For this review, take the finished solid that the model builds, in its own axes (mm). Face numbers are marked on the shaded views. Round coordinates to 2 decimals unless told otherwise and drop trailing zeros. Order: outer loops, then holes, each group sorted by start corner. A loop starts at its lowest first (then second) coordinate and runs counter-clockwise, first axis right, second up. Notation, with made-up numbers: (22, 72.25) - (49, 72.25) arc R12 ccw to (49, 93.25) - close; hole circle Ø4 at (8.5, 84). An arc over 180 degrees is marked (long way). One line per item, written item: value.
```python
from build123d import *

# Parameters (mm, degrees)
SPUR_START             = -54.751290346
SPUR_GEAR_AI_OUTLINE_R = 4.7625
SPUR_GEAR_AI_DEPTH     = 11.684
CUT_EXTRUDE1_DEPTH     = 45.73825268


# Read off the part's stored shape, not the designer's step: spur gear_ai
with BuildPart() as part:
    # spur gear_ai outline → spur gear_ai (new body)
    with BuildSketch(Plane.YZ.offset(SPUR_START)):
        with BuildLine():
            ThreePointArc((6.265843754, 23.742611923), (6.505460201, 24.059955507), (6.73322633, 24.385908852))
            ThreePointArc((6.73322633, 24.385908852), (5.912883536, 25.630805773), (4.677624003, 26.465589895))
            ThreePointArc((4.677624003, 26.465589895), (5.034990844, 27.171459646), (5.320429206, 27.90935402))
            ThreePointArc((5.320429206, 27.90935402), (6.767344667, 27.549956895), (8.241399844, 27.773322024))
            ThreePointArc((8.241399844, 27.773322024), (8.331225097, 28.160690604), (8.40672264, 28.551104632))
            ThreePointArc((8.40672264, 28.551104632), (7.150957012, 29.354711085), (5.682953985, 29.614899012))
            ThreePointArc((5.682953985, 29.614899012), (5.722321747, 30.405097306), (5.682953985, 31.1952956))
            ThreePointArc((5.682953985, 31.1952956), (7.150957012, 31.455483527), (8.40672264, 32.25908998))
            ThreePointArc((8.40672264, 32.25908998), (8.331225097, 32.649504008), (8.241399844, 33.036872588))
            ThreePointArc((8.241399844, 33.036872588), (6.767344667, 33.260237716), (5.320429206, 32.900840592))
            ThreePointArc((5.320429206, 32.900840592), (5.034990844, 33.638734965), (4.677624003, 34.344604716))
            ThreePointArc((4.677624003, 34.344604716), (5.912883536, 35.179388839), (6.73322633, 36.42428576))
            ThreePointArc((6.73322633, 36.42428576), (6.505460201, 36.750239104), (6.265843754, 37.067582688))
            ThreePointArc((6.265843754, 37.067582688), (4.82837656, 36.672084633), (3.652733492, 35.755245485))
            ThreePointArc((3.652733492, 35.755245485), (3.091843894, 36.313247297), (2.478269946, 36.812737212))
            ThreePointArc((2.478269946, 36.812737212), (3.26719839, 38.077775771), (3.510273629, 39.548709173))
            ThreePointArc((3.510273629, 39.548709173), (3.169621747, 39.75384154), (2.821645965, 39.94628854))
            ThreePointArc((2.821645965, 39.94628854), (1.669317892, 39.000312507), (0.968226585, 37.684561153))
            ThreePointArc((0.968226585, 37.684561153), (0.228868656, 37.966186822), (-0.534819889, 38.172930557))
            ThreePointArc((-0.534819889, 38.172930557), (-0.328635429, 39.649486893), (-0.704857663, 41.092119028))
            ThreePointArc((-0.704857663, 41.092119028), (-1.099493493, 41.140961166), (-1.495660434, 41.175235748))
            ThreePointArc((-1.495660434, 41.175235748), (-2.163601395, 39.842349587), (-2.268915885, 38.35519139))
            ThreePointArc((-2.268915885, 38.35519139), (-3.058900442, 38.311745278), (-3.840654895, 38.189994964))
            ThreePointArc((-3.840654895, 38.189994964), (-4.252865586, 39.622759072), (-5.18333305, 40.787645738))
            ThreePointArc((-5.18333305, 40.787645738), (-5.563716707, 40.671752399), (-5.939573945, 40.541928176))
            ThreePointArc((-5.939573945, 40.541928176), (-6.007634734, 39.052600014), (-5.498962575, 37.651178136))
            ThreePointArc((-5.498962575, 37.651178136), (-6.202978253, 37.290172471), (-6.867626169, 36.860979842))
            ThreePointArc((-6.867626169, 36.860979842), (-7.826957037, 38.002213793), (-9.150783454, 38.687935502))
            ThreePointArc((-9.150783454, 38.687935502), (-9.451143149, 38.427345697), (-9.741701553, 38.155870456))
            ThreePointArc((-9.741701553, 38.155870456), (-9.19811384, 36.767618662), (-8.16340907, 35.694251677))
            ThreePointArc((-8.16340907, 35.694251677), (-8.659725162, 35.078107619), (-9.092342877, 34.41568398))
            ThreePointArc((-9.092342877, 34.41568398), (-10.4329169, 35.068058055), (-11.921200656, 35.156047294))
            ThreePointArc((-11.921200656, 35.156047294), (-12.089601468, 34.795819368), (-12.24462085, 34.429633645))
            ThreePointArc((-12.24462085, 34.429633645), (-11.18337589, 33.382499566), (-9.801548363, 32.822782378))
            ThreePointArc((-9.801548363, 32.822782378), (-10.004347308, 32.05803683), (-10.13013129, 31.276921247))
            ThreePointArc((-10.13013129, 31.276921247), (-11.62015104, 31.327634041), (-13.015554353, 30.802676673))
            ThreePointArc((-13.015554353, 30.802676673), (-13.022878253, 30.405097306), (-13.015554353, 30.007517939))
            ThreePointArc((-13.015554353, 30.007517939), (-11.62015104, 29.48256057), (-10.13013129, 29.533273365))
            ThreePointArc((-10.13013129, 29.533273365), (-10.004347308, 28.752157782), (-9.801548363, 27.987412234))
            ThreePointArc((-9.801548363, 27.987412234), (-11.18337589, 27.427695046), (-12.24462085, 26.380560967))
            ThreePointArc((-12.24462085, 26.380560967), (-12.089601468, 26.014375244), (-11.921200656, 25.654147317))
            ThreePointArc((-11.921200656, 25.654147317), (-10.4329169, 25.742136557), (-9.092342877, 26.394510632))
            ThreePointArc((-9.092342877, 26.394510632), (-8.659725162, 25.732086993), (-8.16340907, 25.115942934))
            ThreePointArc((-8.16340907, 25.115942934), (-9.19811384, 24.04257595), (-9.741701553, 22.654324156))
            ThreePointArc((-9.741701553, 22.654324156), (-9.451143149, 22.382848915), (-9.150783454, 22.12225911))
            ThreePointArc((-9.150783454, 22.12225911), (-7.826957037, 22.807980819), (-6.867626169, 23.94921477))
            ThreePointArc((-6.867626169, 23.94921477), (-6.202978253, 23.520022141), (-5.498962575, 23.159016476))
            ThreePointArc((-5.498962575, 23.159016476), (-6.007634734, 21.757594598), (-5.939573945, 20.268266436))
            ThreePointArc((-5.939573945, 20.268266436), (-5.563716707, 20.138442212), (-5.18333305, 20.022548874))
            ThreePointArc((-5.18333305, 20.022548874), (-4.252865586, 21.187435539), (-3.840654895, 22.620199648))
            ThreePointArc((-3.840654895, 22.620199648), (-3.058900442, 22.498449333), (-2.268915885, 22.455003221))
            ThreePointArc((-2.268915885, 22.455003221), (-2.163601395, 20.967845024), (-1.495660434, 19.634958864))
            ThreePointArc((-1.495660434, 19.634958864), (-1.099493492, 19.669233445), (-0.704857663, 19.718075584))
            ThreePointArc((-0.704857663, 19.718075584), (-0.328635429, 21.160707719), (-0.534819889, 22.637264055))
            ThreePointArc((-0.534819889, 22.637264055), (0.228868655, 22.84400779), (0.968226585, 23.125633458))
            ThreePointArc((0.968226585, 23.125633458), (1.669317892, 21.809882105), (2.821645965, 20.863906072))
            ThreePointArc((2.821645965, 20.863906072), (3.169621747, 21.056353072), (3.510273629, 21.261485438))
            ThreePointArc((3.510273629, 21.261485438), (3.26719839, 22.73241884), (2.478269946, 23.997457399))
            ThreePointArc((2.478269946, 23.997457399), (3.091843894, 24.496947314), (3.652733492, 25.054949127))
            ThreePointArc((3.652733492, 25.054949127), (4.82837656, 24.138109979), (6.265843754, 23.742611923))
        make_face()
        with Locations((-2.227878253, 30.405097306)):
            Circle(SPUR_GEAR_AI_OUTLINE_R, mode=Mode.SUBTRACT)
    extrude(amount=SPUR_GEAR_AI_DEPTH)

    # Sketch1 → Cut-Extrude1 (cut, through all)
    with BuildSketch(Plane(origin=(-43.067290346, 0, 0), x_dir=(0, 0, -1), z_dir=(1, 0, 0))):
        Polygon((-27.655466649, 2.534621747), (-33.154727963, 2.534621747), (-35.90435862, -2.227878253), (-33.154727963, -6.990378253), (-27.655466649, -6.990378253), (-24.905835992, -2.227878253), align=None)
    extrude(amount=-CUT_EXTRUDE1_DEPTH, mode=Mode.SUBTRACT)


solid = part.part
```
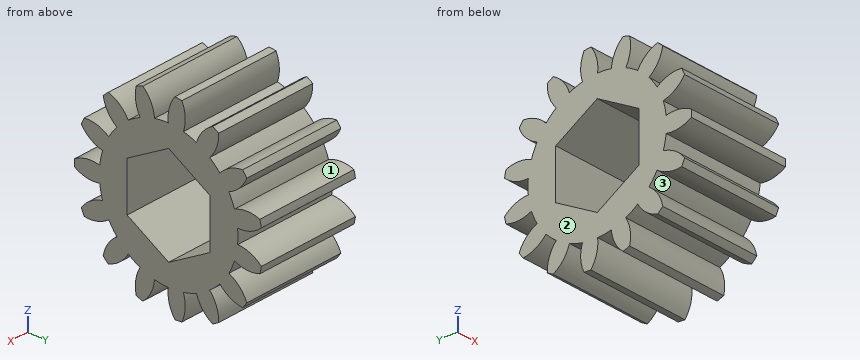
Item 1: Take a section at B-B (y = 2). Write out the cut boundary in (x, z), plus the area to 3 significant figures.
Returned:
outline: (-54.75, 21.46) - (-43.07, 21.46) - (-43.07, 27.35) - (-54.75, 27.35) - close; (-54.75, 33.46) - (-43.07, 33.46) - (-43.07, 39.36) - (-54.75, 39.36) - close
area: 138 mm^2
Item 2: Wall thickness on line 1 (Y direction, x = -54, z = 30.25); line 2 (Z direction, x = -51, y = 5); line 3 (Y direction, x = -47.75, z = 26.5): over which ranges is each line inside the solid? List them lowest first.
Returned:
line 1: -13.02 to -6.99, 2.53 to 5.72
line 2: 24.06 to 26.31, 27.09 to 33.72, 34.5 to 36.75
line 3: -12.16 to -4.99, 0.53 to 4.7
Item 3: The part is to be moulded in two halves that separate along Z. For the marked faces 1, 2 and 3, say which applies: +Z half, -Z half, draft (parallel to the pull), parting line (faces both ways), or undercut.
Returned:
face 1: undercut
face 2: draft
face 3: undercut
Item 4: For P1, Ø5, axis at x = -46.5, z = 34.5, coming from the -Y side; P2, Ø1, axis at x = -44.5, y = -5.5, coming from the +Z side, all flat-tipped, find the tip position at first contact; note any pin that passes through.
Returned:
P1: y = -12.24
P2: z = 40.79
Item 5: Take a section at A-A (z = 39). Write out the cut boundary in (x, y).
Returned:
outline: (-54.75, -6) - (-43.07, -6) - (-43.07, -4) - (-54.75, -4) - close; (-54.75, -2.3) - (-43.07, -2.3) - (-43.07, -0.35) - (-54.75, -0.35) - close; (-54.75, 1.67) - (-43.07, 1.67) - (-43.07, 3.49) - (-54.75, 3.49) - close
